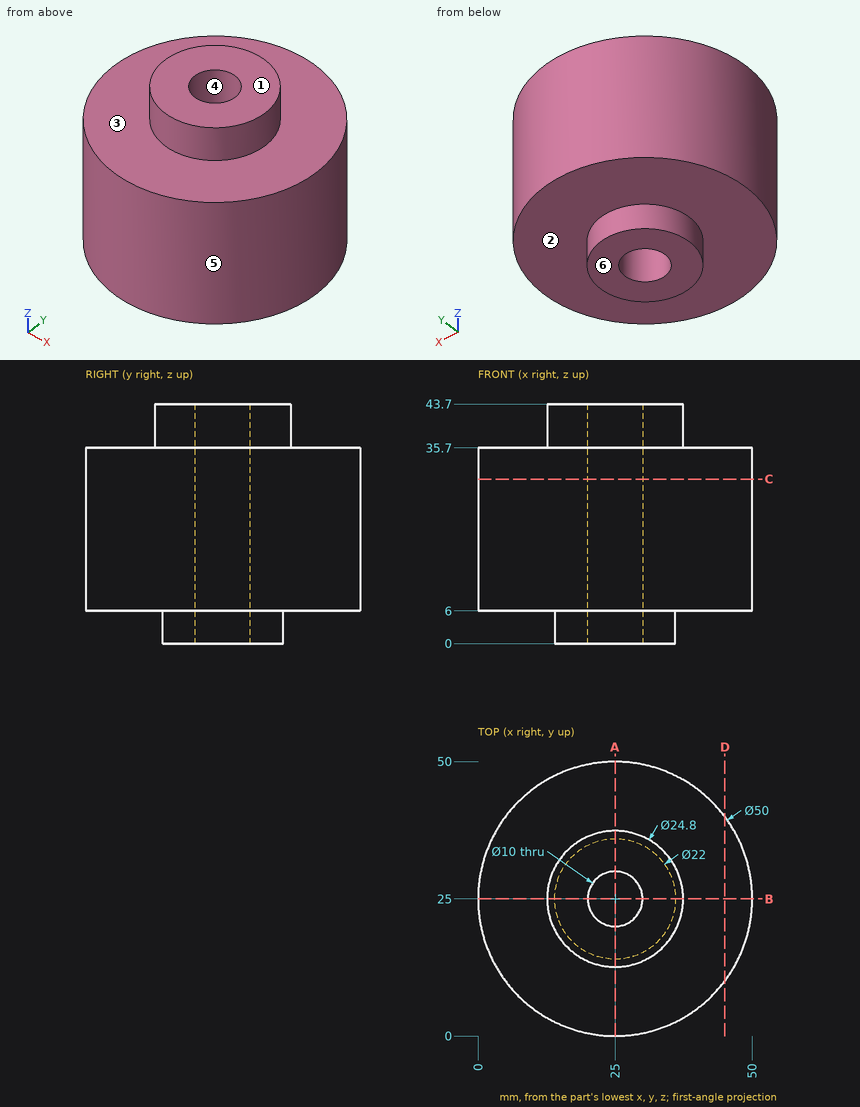
The drawing under review shows one solid part. Ordinate dimensions are in mm from its lowest x, y, z. A direction names the side the tool comes from. Give positions to 0.01 mm unless a question says otherwise; leave off trailing zeros. Write each loop counter-clockwise with the first axis right and the second up, starting at its lowest first coordinate (ties: lowest second). Pieces come first, ordered by that corner, then holes. Notation, with made-up numbers: (-33, 8) -> (10, 8) arc R21 ccw to (10, 39) -> close; hole circle Ø4 at (6, 23). An arc over 180 degrees is marked (long way). Put each result on its own line as item: value.
(1) To check wall thickness, follow probe 1 along Y at (x, z) = (25, 9.5); probe 2 along Z at (x, y) = (32, 11.5); probe 3 along X at (y, z) = (29, 24). State the ranges of each line that lie inside material, in increasing order. Write a range as from..to.
Results are:
probe 1: 0..20, 30..50
probe 2: 6..35.7
probe 3: 0.32..22, 28..49.68
(2) For pin 1 Ø1 at (x, z) = (29, 36.5) entering from +Y; pin 2 Ø1.5 at (x, y) = (20.5, 37) entering from -Z; pin 3 Ø8 at (y, z) = (37.5, 5.5) entering from -X; pin 4 Ø6 at (x, y) = (38, 29) entering from +Z, all flat-tipped, find the tip position at first contact; note any pin that passes through.
Results are:
pin 1: y = 36.9
pin 2: z = 6
pin 3: x = 1.5
pin 4: z = 43.7
(3) We need section D-D, the plane x = 45. Give the boundary of the cut face in (y, z).
Results are:
outline: (10, 6) -> (40, 6) -> (40, 35.7) -> (10, 35.7) -> close
(4) Tool access review of the marked faces 1, 2 and 3: name each direction out of +Z, -Z, +X, -X, +Y, -Y from which nothing blocks a thin tool from reaching the whole face with its end or side.
Results are:
face 1: +Z, +X, -X, +Y, -Y
face 2: -Z
face 3: +Z
(5) The part is to be moulded in two halves that separate along X. For the marked faces 4, 5 and 6, say which applies: pulls with the +X half, pulls with the -X half, needs draft (parallel to the pull), parting line crosses it, or undercut.
Results are:
face 4: undercut
face 5: parting line crosses it
face 6: needs draft
(6) We need section A-A, the plane x = 25. Give the boundary of the cut face in (y, z).
Results are:
outline: (0, 6) -> (14, 6) -> (14, 0) -> (20, 0) -> (20, 43.7) -> (12.6, 43.7) -> (12.6, 35.7) -> (0, 35.7) -> close; (30, 0) -> (36, 0) -> (36, 6) -> (50, 6) -> (50, 35.7) -> (37.4, 35.7) -> (37.4, 43.7) -> (30, 43.7) -> close
(7) We need section C-C, the plane z = 30. Give the boundary of the cut face in (x, y), and give its area (3 significant figures).
Results are:
outline: circle Ø50 at (25, 25); hole circle Ø10 at (25, 25)
area: 1,880 mm²
